Source: CAD feature listing. Evaluate the final solid. Frame: model axes, mm. Give positions to 0.01 mm unless a question says otherwise; leave off trailing zeros. Order: outer loops, then holes, each group sorted by start corner. A loop starts at its lowest first (then second) coordinate and runs counter-clockwise, first axis right, second up. Notation, with made-up numbers: (86, 16) -> (131, 16) arc R20 ccw to (131, 48) -> close; hole circle Ø2 at (-34, -37.5). An arc over 180 degrees is marked (long way). Answer in a Markdown table with one row per item.
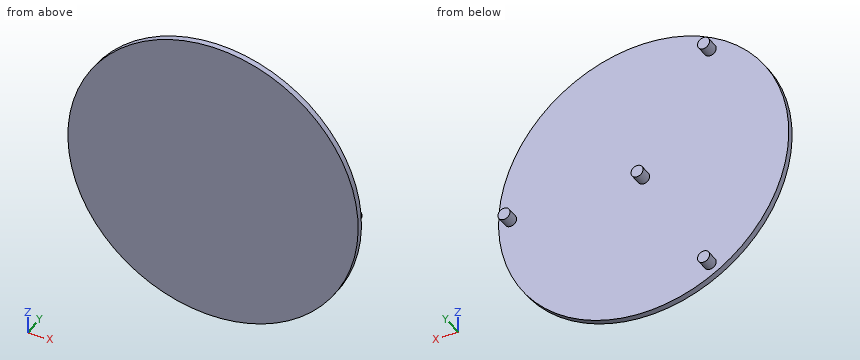
```python
from build123d import *

# Parameters (mm, degrees)
SKETCH1_R           = 76.2
BOSS_EXTRUDE1_DEPTH = 3.175
SKETCH3_R           = 3.175
BOSS_EXTRUDE2_DEPTH = 6.35
CIRPATTERN1_COUNT   = 3


with BuildPart() as part:
    # Sketch1 → Boss-Extrude1 (new body)
    with BuildSketch(Plane(origin=(0, 0, 0), x_dir=(1, 0, 0), z_dir=(0, 1, 0))):
        with Locations(Location((0, 0, 0), (0, 0, 270))):
            Circle(SKETCH1_R)
    extrude(amount=BOSS_EXTRUDE1_DEPTH)

    # Sketch3 → Boss-Extrude2 (add)
    with BuildSketch(Plane(origin=(0, 3.175, 0), x_dir=(1, 0, 0), z_dir=(0, 1, 0))):
        with Locations(Location((0, 0, 0), (0, 0, 270))):
            Circle(SKETCH3_R)
        with Locations(Location((69.85, 0, 0), (0, 0, 270))):
            Circle(SKETCH3_R)
    boss_extrude2 = extrude(amount=BOSS_EXTRUDE2_DEPTH)

    # CirPattern1: Boss-Extrude2 ×3 about axis
    cirpattern1_axis = Axis((0, 0, 0), (0, 1, 0))
    for i in range(1, CIRPATTERN1_COUNT):
        add(boss_extrude2.rotate(cirpattern1_axis, i * 360 / CIRPATTERN1_COUNT))


solid = part.part
```
(1) Ray query, probe 1 along Y at (x, z) = (55.5, 6.5) (3 decimals); probe 2 along X at (y, z) = (7.75, 0.5); probe 3 along Z at (x, y) = (-25, 3). Return the intervals inside material, ascending.
A:
| item | result |
|---|---|
| probe 1 | y = 0 to 3.175 |
| probe 2 | x = -3.14 to 3.14, 66.71 to 72.99 |
| probe 3 | z = -71.98 to 71.98 |
(2) Section query C-C (y = 7.75). Return the cut outline in (x, z) (3 decimals), plus the area to 3 significant figures.
A:
| item | result |
|---|---|
| outline | circle Ø6.35 at (-34.925, -60.492); circle Ø6.35 at (-34.925, 60.492); circle Ø6.35 at (0, 0); circle Ø6.35 at (69.85, 0) |
| area | 127 mm^2 |
(3) First-contact query: pin 1 Ø4 at (x, z) = (-51.5, -6) entering from +Y (3 decimals); pin 2 Ø3 at (x, y) = (58, 5) entering from +Z. Flat tips, straight axial feed; report the tip coordinate or a pass-through.
A:
| item | result |
|---|---|
| pin 1 | stops at y = 3.175 |
| pin 2 | passes through |
(4) Section query B-B (x = 69.85). Return the cut outline in (y, z) (3 decimals), plus the area to 3 significant figures.
A:
| item | result |
|---|---|
| outline | (0, -30.454) -> (3.175, -30.454) -> (3.175, -3.175) -> (9.525, -3.175) -> (9.525, 3.175) -> (3.175, 3.175) -> (3.175, 30.454) -> (0, 30.454) -> close |
| area | 234 mm^2 |
(5) Section query A-A (z = 0). Return the cut outline in (x, y) (3 decimals).
A:
| item | result |
|---|---|
| outline | (-76.2, 0) -> (76.2, 0) -> (76.2, 3.175) -> (73.025, 3.175) -> (73.025, 9.525) -> (66.675, 9.525) -> (66.675, 3.175) -> (3.175, 3.175) -> (3.175, 9.525) -> (-3.175, 9.525) -> (-3.175, 3.175) -> (-76.2, 3.175) -> close |
(6) Section query D-D (x = 0). Return the cut outline in (y, z) (3 decimals).
A:
| item | result |
|---|---|
| outline | (0, -76.2) -> (3.175, -76.2) -> (3.175, -3.175) -> (9.525, -3.175) -> (9.525, 3.175) -> (3.175, 3.175) -> (3.175, 76.2) -> (0, 76.2) -> close |
